from build123d import *

# Parameters (mm, degrees)
EXTRUDE_1_DEPTH      = 49
SKETCH_3_R           = 1.5
CUT_EXTRUDE_1_DEPTH  = 64.718207759
EXTRUDE_3_DEPTH      = 3.5
EXTRUDE_4_DEPTH      = 3.5
EXTRUDE_5_DEPTH      = 1.5
EXTRUDE_5_DEPTH_BACK = 1.5
SKETCH_8_R           = 2
CUT_EXTRUDE_2_DEPTH  = 10
CUT_EXTRUDE_3_REACH  = 67.146
EXTRUDE_6_DEPTH      = 3.5
SKETCH_11_R          = 1.6
CUT_EXTRUDE_4_DEPTH  = 10


with BuildPart() as part:
    # 草图1 → 凸台-拉伸1 (new body)
    with BuildSketch(Plane(origin=(0, 0, 0), x_dir=(0, 0, -1), z_dir=(1, 0, 0))):
        Polygon((0, 0), (0, 25), (4, 25), (4, 4), (34.9, 4), (34.9, 0), align=None)
    extrude(amount=EXTRUDE_1_DEPTH)

    # 草图3 → 切除-拉伸1 (cut, through all)
    with BuildSketch(Plane(origin=(0, 4, 0), x_dir=(1, 0, 0), z_dir=(0, 1, 0))):
        with Locations(Location((20.5, 32.05, 0), (0, 0, 270))):
            Circle(SKETCH_3_R)
        with Locations(Location((28.5, 32.05, 0), (0, 0, 90))):
            Circle(SKETCH_3_R)
        with Locations(Location((42.5, 15.55, 0), (0, 0, 270))):
            Circle(SKETCH_3_R)
        with Locations(Location((6.5, 15.55, 0), (0, 0, 90))):
            Circle(SKETCH_3_R)
        with Locations(Location((29.5, 8.55, 0), (0, 0, 270))):
            Circle(SKETCH_3_R)
        with Locations(Location((19.5, 8.55, 0), (0, 0, 90))):
            Circle(SKETCH_3_R)
        Polygon((31.5, 34.9), (45.5, 20.05), (49, 20.05), (49, 34.9), align=None)
        Polygon((0, 20.05), (0, 34.9), (17.5, 34.9), (3.5, 20.05), align=None)
    extrude(amount=-CUT_EXTRUDE_1_DEPTH, mode=Mode.SUBTRACT)

    # 草图5 → 凸台-拉伸3 (add)
    with BuildSketch(Plane(origin=(49, 0, 0), x_dir=(0, 0, -1), z_dir=(1, 0, 0))):
        Polygon((20.05, 0), (20.05, 4), (4, 25), (0, 25), (0, 0), align=None)
    extrude(amount=-EXTRUDE_3_DEPTH)

    # 草图6 → 凸台-拉伸4 (add)
    with BuildSketch(Plane.ZY):
        Polygon((-4, 25), (0, 25), (0, 0), (-20.05, 0), (-20.05, 4), align=None)
    extrude(amount=-EXTRUDE_4_DEPTH)

    # 草图7 → 凸台-拉伸5 (add, two sides: drawn at the far end of the back side and taken through both)
    with BuildSketch(Plane(origin=(24.5, 0, 0), x_dir=(0, 0, -1), z_dir=(1, 0, 0)).offset(-EXTRUDE_5_DEPTH_BACK)):
        Polygon((34.9, 4), (34.9, 0), (0, 0), (0, 25), (4, 25), align=None)
    extrude(amount=EXTRUDE_5_DEPTH + EXTRUDE_5_DEPTH_BACK)

    # 草图8 → 切除-拉伸2 (cut)
    with BuildSketch(Plane(origin=(0, 0, -4), x_dir=(-1, 0, 0), z_dir=(0, 0, -1))):
        with Locations(Location((-8.5, 21.5, 0), (0, 0, 90))):
            Circle(SKETCH_8_R)
        with Locations(Location((-8.5, 10.5, 0), (0, 0, 90))):
            Circle(SKETCH_8_R)
        with Locations(Location((-40.5, 10.5, 0), (0, 0, 90))):
            Circle(SKETCH_8_R)
        with Locations(Location((-40.5, 21.5, 0), (0, 0, 90))):
            Circle(SKETCH_8_R)
    extrude(amount=-CUT_EXTRUDE_2_DEPTH, mode=Mode.SUBTRACT)

    # 切除-拉伸3: up to this face of the body (flat: up to its plane)
    cut_extrude_3_end = Plane(part.part.faces().sort_by_distance((34.743076347, 4, -17.196256648))[0])
    # 草图9 → 切除-拉伸3 (cut, up to the picked face)
    with BuildSketch(Plane(origin=(0, 25, 0), x_dir=(1, 0, 0), z_dir=(0, 1, 0)), mode=Mode.PRIVATE) as cut_extrude_3_sk1:
        with BuildLine():
            Line((26, 33.310952021), (26, 30.789047979))
            ThreePointArc((26, 30.789047979), (25.7, 32.05), (26, 33.310952021))
        make_face()
    cut_extrude_3_tool1 = split(extrude(cut_extrude_3_sk1.sketch, amount=-CUT_EXTRUDE_3_REACH, mode=Mode.PRIVATE), bisect_by=cut_extrude_3_end, keep=Keep.BOTH, mode=Mode.PRIVATE)
    # 草图9 → 切除-拉伸3 (cut, up to the picked face)
    with BuildSketch(Plane(origin=(0, 25, 0), x_dir=(1, 0, 0), z_dir=(0, 1, 0)), mode=Mode.PRIVATE) as cut_extrude_3_sk2:
        with BuildLine():
            Line((23, 33.310952021), (23, 30.789047979))
            ThreePointArc((23, 30.789047979), (23.3, 32.05), (23, 33.310952021))
        make_face()
    cut_extrude_3_tool2 = split(extrude(cut_extrude_3_sk2.sketch, amount=-CUT_EXTRUDE_3_REACH, mode=Mode.PRIVATE), bisect_by=cut_extrude_3_end, keep=Keep.BOTH, mode=Mode.PRIVATE)
    add(cut_extrude_3_tool1.solids().sort_by(Axis((25.879431, 25, -32.05), (0, -1, 0)))[0], mode=Mode.SUBTRACT)
    add(cut_extrude_3_tool2.solids().sort_by(Axis((23.120569, 25, -32.05), (0, -1, 0)))[0], mode=Mode.SUBTRACT)

    # 草图10 → 凸台-拉伸6 (add)
    with BuildSketch(Plane(origin=(3.5, 0, 0), x_dir=(0, 0, -1), z_dir=(1, 0, 0))):
        Polygon((20.05, 4), (4, 25), (20.05, 25), align=None)
    extrude(amount=-EXTRUDE_6_DEPTH)

    # 草图11 → 切除-拉伸4 (cut)
    with BuildSketch(Plane.ZY):
        with Locations((-8.05, 15)):
            Circle(SKETCH_11_R)
        with Locations((-16.05, 15)):
            Circle(SKETCH_11_R)
    extrude(amount=-CUT_EXTRUDE_4_DEPTH, mode=Mode.SUBTRACT)


solid = part.part
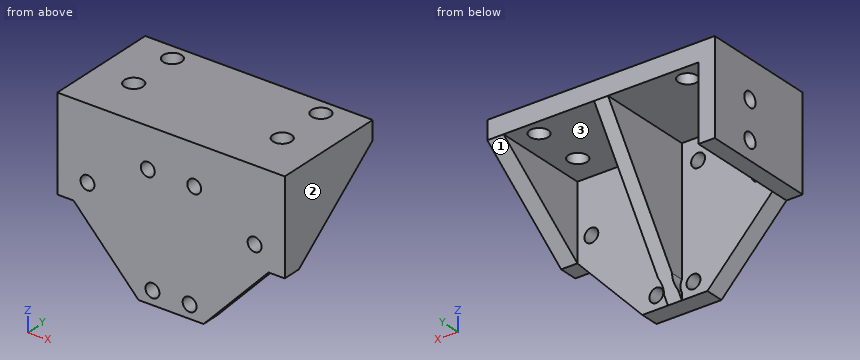
Design review of the part built by this model. Coordinates are the model's own, in mm. Face numbers are marked on the shaded views. A direction names the side the tool comes from. Round coordinates to 2 decimals unless told otherwise and drop trailing zeros. Loops run counter-clockwise (first coordinate to the right, second up) from the corner with the lowest first, then second, coordinate; pieces in that order, holes last. Notation, with made-up numbers: (-7.75, 54.25) - (2.25, 54.25) arc R10 cw to (2.25, 70.25) - close; hole circle Ø2 at (87.25, 22). An arc over 180 degrees is marked (long way). One line per question, with ' | ' between items.
1. Clearance check with flat-ended pins moving along their axes: P1, Ø2.5, axis at x = 19.5, z = -8.55, coming from the +Y side; P2, Ø6, axis at x = 10, z = -14.5, coming from the +Y side; P3, Ø6, axis at x = 31, y = 15.5, coming from the -Z side; P4, Ø4, axis at x = 23, y = 12, coming from the -Z side. State where each tip first meets the part, or that it passes through.
Results are:
P1: passes through | P2: stops at y = 4 | P3: stops at z = -4 | P4: stops at z = -26.07
2. For the marked faces 1, 2 and 3, list the 3-axis set-ups (+Z, -Z, +X, -X, +Y, -Y) from which the entire face can be reached by the end or side of a thin tool; tool diameter is ignored.
Results are:
face 1: -Z, +X, +Y | face 2: +Z, -Z, +X, +Y, -Y | face 3: -Z, +Y
3. We need section C-C, the plane y = 2.25. State the section outline as (x, z) points.
Results are:
outline: (0, -20.05) - (3.5, -20.05) - (17.5, -34.9) - (31.5, -34.9) - (45.5, -20.05) - (49, -20.05) - (49, 0) - (0, 0) - close; hole circle Ø3 at (6.5, -15.55); hole circle Ø3 at (19.5, -8.55); hole circle Ø3 at (20.5, -32.05); hole circle Ø3 at (28.5, -32.05); hole circle Ø3 at (29.5, -8.55); hole circle Ø3 at (42.5, -15.55)
4. We need section B-B, the plane y = 10.5. State the section outline as (x, z) points, and give its area (3 significant figures).
Results are:
outline: (0, -20.05) - (3.5, -20.05) - (3.5, -4) - (6.5, -4) - (6.5, 0) - (0, 0) - close; (10.5, -4) - (23, -4) - (23, -25.34) - (26, -25.34) - (26, -4) - (38.5, -4) - (38.5, 0) - (10.5, 0) - close; (42.5, -4) - (45.5, -4) - (45.5, -15.08) - (49, -15.08) - (49, 0) - (42.5, 0) - close | area: 323 mm²
5. We need section D-D, the plane z = -32.05. State the section outline as (x, y) points.
Results are:
outline: (14.81, 0) - (19, 0) - (19, 4) - (14.81, 4) - close; (22, 0) - (27, 0) - (27, 4) - (25.7, 4) - (25.7, 5.94) - (23.3, 5.94) - (23.3, 4) - (22, 4) - close; (30, 0) - (34.19, 0) - (34.19, 4) - (30, 4) - close
6. For L1, parallel to X at y = 10.5, z = -1.6; L2, parallel to X at y = 1.45, z = -15.55; L3, parallel to Z at x = 28.5, y = 1.6, list the stretches that pass through material, from the lowest coordinate up. Write a range as [from, to].
Results are:
L1: x = [0, 6.5], [10.5, 38.5], [42.5, 49] | L2: x = [0, 5], [8, 41], [44, 49] | L3: z = [-34.9, -33.55], [-30.55, -9.67], [-7.43, 0]
7. We need section A-A, the plane z = -15.55. State the section outline as (x, y) points, and give its area (3 significant figures).
Results are:
outline: (0, 0) - (5, 0) - (5, 4) - (3.5, 4) - (3.5, 13.48) - (0, 13.48) - close; (0, 16.52) - (3.5, 16.52) - (3.5, 25) - (0, 25) - close; (8, 0) - (41, 0) - (41, 4) - (26, 4) - (26, 17.15) - (23, 17.15) - (23, 4) - (8, 4) - close; (44, 0) - (49, 0) - (49, 9.89) - (45.5, 9.89) - (45.5, 4) - (44, 4) - close | area: 295 mm²
